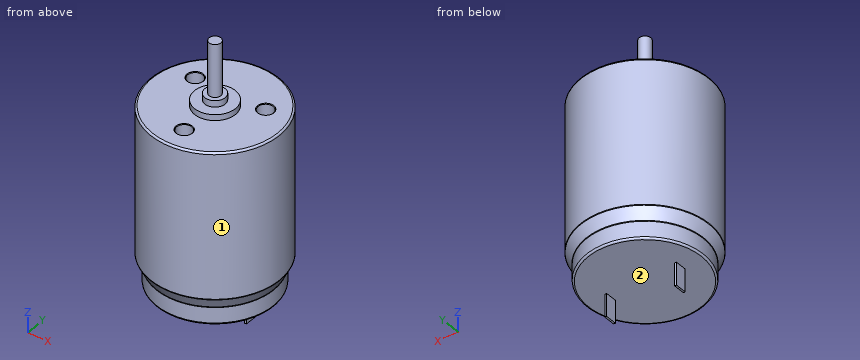
from build123d import *

# Parameters (mm, degrees)
SKETCH1_R           = 11
BOSS_EXTRUDE1_DEPTH = 25
SKETCH2_R           = 10
SKETCH3_R           = 10
BOSS_EXTRUDE2_DEPTH = 3
SKETCH4_R           = 1.3
CUT_EXTRUDE1_DEPTH  = 5
CHAMFER1_SIZE       = 0.1
SKETCH5_R           = 3.5
BOSS_EXTRUDE3_DEPTH = 1
SKETCH6_R           = 1.75
BOSS_EXTRUDE4_DEPTH = 1.1
SKETCH7_R           = 1
BOSS_EXTRUDE5_DEPTH = 9
SKETCH8_W           = 0.3
SKETCH8_H           = 2
BOSS_EXTRUDE6_DEPTH = 3.9
FILLET1_R           = 0.3


with BuildPart() as part:
    # Sketch1 → Boss-Extrude1 (new body)
    with BuildSketch(Plane.XY):
        Circle(SKETCH1_R)
    extrude(amount=-BOSS_EXTRUDE1_DEPTH)

    # Sketch2 → section 1 of loft1
    with BuildSketch(Plane(origin=(0, 0, -27), x_dir=(-1, 0, 0), z_dir=(0, 0, -1)), mode=Mode.PRIVATE) as loft1_s1:
        Circle(SKETCH2_R)
    # loft from a face of the part (loft1)
    loft([part.faces().sort_by_distance((0, 0, -25))[0], loft1_s1.sketch])

    # Sketch3 → Boss-Extrude2 (add)
    with BuildSketch(Plane(origin=(0, 0, -27), x_dir=(-1, 0, 0), z_dir=(0, 0, -1))):
        Circle(SKETCH3_R)
    extrude(amount=BOSS_EXTRUDE2_DEPTH)

    # Sketch4 → Cut-Extrude1 (cut)
    with BuildSketch(Plane.XY):
        with Locations((-6.062177826, 3.5)):
            Circle(SKETCH4_R)
        with Locations((6.062177826, 3.5)):
            Circle(SKETCH4_R)
        with Locations((0, -7)):
            Circle(SKETCH4_R)
    extrude(amount=-CUT_EXTRUDE1_DEPTH, mode=Mode.SUBTRACT)

    # Chamfer1
    chamfer1_edges = [part.edges().sort_by_distance(p)[0] for p in [
        (-7.362177826, 3.5, 0),
        (4.762177826, 3.5, 0),
        (-1.3, -7, 0),
    ]]
    chamfer(chamfer1_edges, length=CHAMFER1_SIZE)

    # Sketch5 → Boss-Extrude3 (add)
    with BuildSketch(Plane.XY):
        Circle(SKETCH5_R)
    extrude(amount=BOSS_EXTRUDE3_DEPTH)

    # Sketch6 → Boss-Extrude4 (add)
    with BuildSketch(Plane.XY.offset(1)):
        Circle(SKETCH6_R)
    extrude(amount=BOSS_EXTRUDE4_DEPTH)

    # Sketch7 → Boss-Extrude5 (add)
    with BuildSketch(Plane.XY.offset(2.1)):
        Circle(SKETCH7_R)
    extrude(amount=BOSS_EXTRUDE5_DEPTH)

    # Sketch8 → Boss-Extrude6 (add)
    with BuildSketch(Plane(origin=(0, 0, -30), x_dir=(-1, 0, 0), z_dir=(0, 0, -1))):
        with Locations((-6, 0)):
            Rectangle(SKETCH8_W, SKETCH8_H)
        with Locations((6, 0)):
            Rectangle(SKETCH8_W, SKETCH8_H)
    extrude(amount=BOSS_EXTRUDE6_DEPTH)

    # Fillet1
    fillet1_edges = [part.edges().sort_by_distance(p)[0] for p in [
        (10, 0, -30),
        (-11, 0, 0),
        (0, 10, -27),
        (-11, 0, -25),
    ]]
    fillet(fillet1_edges, radius=FILLET1_R)


solid = part.part
Could you check a few things on this model? Use its own coordinates, in mm. Face numbers are marked on the shaded views. Round coordinates to 2 decimals unless told otherwise and drop trailing zeros. Write each loop counter-clockwise with the first axis right and the second up, starting at its lowest first coordinate (ties: lowest second). Pieces come first, ordered by that corner, then holes. Notation, with made-up numbers: (22.5, -18) - (39.5, -18) arc R18 cw to (39.5, 14) - close; hole circle Ø4 at (18.25, 15.5). An arc over 180 degrees is marked (long way). Use a Markdown table: item, result.
Q1. For pin 1 (1.5 mm diameter, centred on y = -1.5, z = -5.5, fed in from +X); pin 2 (5 mm diameter, centred on x = 8, y = -4, fed in from -Z); pin 3 (0.6 mm diameter, centred on y = 0, z = -32, fed in from +X), each with a flat end and sliding along its axis, tell me the tip position at first contact or that it passes through.
Output values:
| item | result |
|---|---|
| pin 1 | x = 10.97 |
| pin 2 | z = -30 |
| pin 3 | x = 6.15 |
Q2. I want a section at A-A (z = -4). List the corners of the cut face in (x, y) for me.
Output values:
| item | result |
|---|---|
| outline | circle Ø22 at (0, 0); hole circle Ø2.6 at (-6.06, 3.5); hole circle Ø2.6 at (0, -7); hole circle Ø2.6 at (6.06, 3.5) |
Q3. Thinking about a two-plate mould opening in Y: for the marked faces 1 and 2, which applies, released by +Y, released by -Y, zero draft, split by the parting line, or undercut?
Output values:
| item | result |
|---|---|
| face 1 | split by the parting line |
| face 2 | zero draft |
Q4. Please list where these lines run through material, in increasing order: L1, parallel to Z at x = 5.5, y = 2.75; L2, parallel to Z at x = 6.75, y = 6; L3, parallel to Y at x = -2.5, z = -10.
Output values:
| item | result |
|---|---|
| L1 | -30 to -5 |
| L2 | -30 to 0 |
| L3 | -10.71 to 10.71 |
Q5. I want a section at B-B (z = -20). List the corners of the cut face in (x, y) for me.
Output values:
| item | result |
|---|---|
| outline | circle Ø22 at (0, 0) |
